Design review of the part built by this model. Coordinates are the model's own, in mm. A direction names the side the tool comes from. Coordinates: 2 decimals unless noted, no trailing zeros. Write each loop counter-clockwise with the first axis right and the second up, starting at its lowest first coordinate (ties: lowest second). Pieces come first, ordered by that corner, then holes. Notation, with made-up numbers: (82, -25.75) - (117, -25.75) arc R17 ccw to (117, -16.75) - close; hole circle Ø7 at (67, 15). An arc over 180 degrees is marked (long way). One line per item, written item: value.
from build123d import *


with BuildPart() as part:
    # 草图1 → 旋转1 (revolve)
    with BuildSketch(Plane.XY):
        Polygon((-185, 25), (185, 25), (185, 7.5), (225, 7.5), (225, 0), (-225, 0), (-225, 7.5), (-185, 7.5), align=None)
    revolve(axis=Axis((-225, 0, 0), (1, 0, 0)))

    # 草图3 → M5 螺纹孔1 (revolve, cut)
    with BuildSketch(Plane(origin=(-215, -7.5, 0), x_dir=(0, 0, -1), z_dir=(1, 0, 0))):
        Polygon((0, 0), (0, 51.2618073), (2.1, 50), (2.1, 0), align=None)
    hole_wizard_m5_1 = revolve(axis=Axis((-215, -13.85, 0), (0, 1, 0)), mode=Mode.SUBTRACT)

    # 镜向1: M5 螺纹孔1 across plane
    add(hole_wizard_m5_1.mirror(Plane(origin=(0, 0, 0), x_dir=(0, 0, 1), z_dir=(1, 0, 0))), mode=Mode.SUBTRACT)


solid = part.part
1. Consider section D-D, the plane y = -17. Write out the cut boundary in (x, z).
Answer block:
outline: (-185, -18.33) - (185, -18.33) - (185, 18.33) - (-185, 18.33) - close
2. Consider section B-B, the plane x = -19. Write out the cut boundary in (y, z).
Answer block:
outline: circle Ø50 at (0, 0)
3. Wall thickness on line 1 along X through (y, z) = (3.5, 0); line 2 along Z through (x, y) = (215, 1); line 3 along Z through (x, y) = (215, 0): over which ranges is each line inside the solid? List them lowest first.
Answer block:
line 1: x = -225 to -217.1, -212.9 to 212.9, 217.1 to 225
line 2: z = -7.43 to -2.1, 2.1 to 7.43
line 3: z = -7.5 to -2.1, 2.1 to 7.5
4. For faces 1 (the face through (-185, -5, 6)), 2 (the face through (205.28, 6.93, -2.87)), 3 (the face through (225, 0, 0)), list the 3-axis set-ups (+Z, -Z, +X, -X, +Y, -Y) from which the entire face can be reached by the end or side of a thin tool; tool diameter is ignored.
Answer block:
face 1: -X
face 2: +X
face 3: +Z, -Z, +X, +Y, -Y
5. Insertion check: pin 1 Ø1 at (x, y) = (51, -12) entering from -Z; pin 2 Ø12 at (y, z) = (-15.5, -18.5) entering from -X; pin 3 Ø2 at (x, y) = (-113, -10) entering from -Z; pin 4 Ø3.5 at (x, z) = (215, 0) entering from +Y. Each pin has a flat end and moves straight along its axis. Give the tip position at first contact, or say it passes through.
Answer block:
pin 1: stops at z = -22.2
pin 2: stops at x = -185
pin 3: stops at z = -23.32
pin 4: passes through
6. Consider section C-C, the plane z = 20. Write out the cut boundary in (x, y).
Answer block:
outline: (-185, -15) - (185, -15) - (185, 15) - (-185, 15) - close
7. Consider section A-A, the plane y = 0. Write out the cut boundary in (x, z).
Answer block:
outline: (-225, -7.5) - (-185, -7.5) - (-185, -25) - (185, -25) - (185, -7.5) - (225, -7.5) - (225, 7.5) - (185, 7.5) - (185, 25) - (-185, 25) - (-185, 7.5) - (-225, 7.5) - close; hole circle Ø4.2 at (-215, 0); hole circle Ø4.2 at (215, 0)
